```python
from build123d import *

# Parameters (mm, degrees)
F1_DEPTH = 1.905
F3_DEPTH = 1.905
F4_R     = 1.8415
F5_R     = 2.413
F6_DEPTH = 1.8415
F7_R     = 1.778
F8_W     = 81.534
F8_H     = 1.905
F9_DEPTH = 25.4
F10_R    = 5.08


with BuildPart() as f1:
    # F0 (on Top) → F1 (new body)
    with BuildSketch(Plane.XY):
        with BuildLine():
            Line((44.45, -15.875), (44.45, 15.875))
            Line((44.45, 15.875), (-44.45, 15.875))
            Line((-44.45, 15.875), (-44.45, -15.875))
            Line((-44.45, -15.875), (-25.4, -15.875))
            ThreePointArc((-25.4, -15.875), (-16.4197438789, -19.5947438789), (-12.7, -28.575))
            Line((-12.7, -28.575), (-12.7, -47.625))
            ThreePointArc((-12.7, -47.625), (0, -60.325), (12.7, -47.625))
            Line((12.7, -47.625), (12.7, -28.575))
            ThreePointArc((12.7, -28.575), (16.4197438789, -19.5947438789), (25.4, -15.875))
            Line((25.4, -15.875), (44.45, -15.875))
        make_face()
        with BuildLine():
            Line((5.1562, -22.3163515329), (5.1562, -47.625))
            ThreePointArc((5.1562, -47.625), (0, -52.7812), (-5.1562, -47.625))
            Line((-5.1562, -47.625), (-5.1562, -22.3163515329))
            ThreePointArc((-5.1562, -22.3163515329), (0, -17.1601515329), (5.1562, -22.3163515329))
        make_face(mode=Mode.SUBTRACT)
    extrude(amount=F1_DEPTH)

    # F2 (on face) → F3 (join)
    with BuildSketch(Plane(origin=(-44.45, 0, 0), x_dir=(0, -1, 0), z_dir=(-1, 0, 0))):
        with BuildLine():
            Line((-15.875, 41.275), (-15.875, 1.905))
            Line((-15.875, 1.905), (15.875, 1.905))
            Line((15.875, 1.905), (15.875, 41.275))
            Line((15.875, 41.275), (12.573, 41.275))
            ThreePointArc((12.573, 41.275), (5.5897728619, 30.0129056853), (-7.6027366345, 31.2610734641))
            ThreePointArc((-7.6027366345, 31.2610734641), (-8.0654902519, 34.6420492241), (-4.6845144919, 35.1048028415))
            ThreePointArc((-4.6845144919, 35.1048028415), (3.4442034806, 34.3357297657), (7.747, 41.275))
            Line((7.747, 41.275), (2.413, 41.275))
            ThreePointArc((2.413, 41.275), (0, 38.862), (-2.413, 41.275))
            Line((-2.413, 41.275), (-7.9572815939, 41.275))
            ThreePointArc((-7.9572815939, 41.275), (-10.0990117962, 39.9735577991), (-12.2407419985, 41.275))
            Line((-12.2407419985, 41.275), (-15.875, 41.275))
        make_face()
        with BuildLine():
            ThreePointArc((15.875, 41.275), (0, 57.15), (-15.875, 41.275))
            Line((-15.875, 41.275), (-12.2407419985, 41.275))
            ThreePointArc((-12.2407419985, 41.275), (-12.4710349135, 41.9437538571), (-12.4975270978, 42.6505527763))
            ThreePointArc((-12.4975270978, 42.6505527763), (-5.5381580453, 52.56256548), (6.5600004581, 52.0009835442))
            ThreePointArc((6.5600004581, 52.0009835442), (7.3595325655, 48.6834714629), (4.0420204843, 47.8839393555))
            ThreePointArc((4.0420204843, 47.8839393555), (-3.4124004118, 48.2299645887), (-7.7004964946, 42.1225628218))
            ThreePointArc((-7.7004964946, 42.1225628218), (-7.7896724982, 41.6869000206), (-7.9572815939, 41.275))
            Line((-7.9572815939, 41.275), (-2.413, 41.275))
            ThreePointArc((-2.413, 41.275), (0, 43.688), (2.413, 41.275))
            Line((2.413, 41.275), (7.747, 41.275))
            ThreePointArc((7.747, 41.275), (7.7353653871, 41.6994188123), (7.7004964946, 42.1225628218))
            ThreePointArc((7.7004964946, 42.1225628218), (9.8350168189, 44.7850731007), (12.4975270978, 42.6505527763))
            ThreePointArc((12.4975270978, 42.6505527763), (12.5541175954, 41.9638108593), (12.573, 41.275))
            Line((12.573, 41.275), (15.875, 41.275))
        make_face()
    extrude(amount=-F3_DEPTH)

    # F4
    f4_edges = [f1.edges().sort_by_distance(p)[0] for p in [
        (-44.45, 0, 0),
        (-42.545, 0, 1.905),
    ]]
    fillet(f4_edges, radius=F4_R)

    # F5 (on face) → F6 (join)
    with BuildSketch(Plane.YZ.offset(44.45)):
        with BuildLine():
            Line((-15.875, 41.3385), (-15.875, 1.905))
            Line((-15.875, 1.905), (-15.875, 0))
            Line((-15.875, 0), (15.875, 0))
            Line((15.875, 0), (15.875, 1.905))
            Line((15.875, 1.905), (15.875, 41.3385))
            ThreePointArc((15.875, 41.3385), (0, 57.2135), (-15.875, 41.3385))
        make_face()
        with BuildLine():
            ThreePointArc((-7.7672171262, 42.0276193774), (-3.8210671013, 34.5402395867), (4.6265424964, 35.0606704009))
            ThreePointArc((4.6265424964, 35.0606704009), (8.0006043661, 34.5499410208), (7.4898749861, 31.1758791512))
            ThreePointArc((7.4898749861, 31.1758791512), (-6.1858969034, 30.3333576051), (-12.5742896147, 42.4546206538))
            ThreePointArc((-12.5742896147, 42.4546206538), (-9.9572527322, 44.6446562598), (-7.7672171262, 42.0276193774))
        make_face(mode=Mode.SUBTRACT)
        with Locations((0, 41.3376752096)):
            Circle(F5_R, mode=Mode.SUBTRACT)
        with BuildLine():
            ThreePointArc((-6.3605039749, 52.2420007561), (5.8932381714, 52.5014590796), (12.591700736, 42.2373412666))
            ThreePointArc((12.591700736, 42.2373412666), (10.3568047712, 39.6585085798), (7.7779720844, 41.8934045446))
            ThreePointArc((7.7779720844, 41.8934045446), (3.6402899771, 48.2336141393), (-3.9289229785, 48.0733451146))
            ThreePointArc((-3.9289229785, 48.0733451146), (-7.2290412974, 48.9418824372), (-6.3605039749, 52.2420007561))
        make_face(mode=Mode.SUBTRACT)
    extrude(amount=-F6_DEPTH)

    # F7
    f7_edges = [f1.edges().sort_by_distance(p)[0] for p in [
        (44.45, 0, 0),
        (42.6085, 0, 1.905),
    ]]
    fillet(f7_edges, radius=F7_R)

    # F8 (on face) → F9 (join)
    with BuildSketch(Plane(origin=(0, 15.875, 0), x_dir=(-1, 0, 0), z_dir=(0, 1, 0))):
        with Locations((-0.0635, 0.9525)):
            Rectangle(F8_W, F8_H)
    extrude(amount=F9_DEPTH)

    # F10
    f10_edges = [f1.edges().sort_by_distance(p)[0] for p in [
        (40.8305, 41.275, 0.9525),
        (-40.7035, 41.275, 0.9525),
    ]]
    fillet(f10_edges, radius=F10_R)


solid = f1.part
```
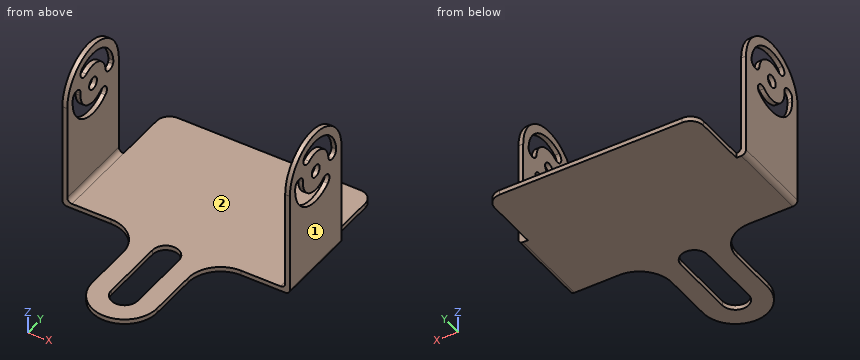
Check sheet for the modelled part. Datum: model origin and axes. Units: mm. Face numbers are marked on the shaded views. A direction names the side the tool comes from. Give positions to 0.01 mm unless a question says otherwise; leave off trailing zeros. Order: outer loops, then holes, each group sorted by start corner. A loop starts at its lowest first (then second) coordinate and runs counter-clockwise, first axis right, second up. Notation, with made-up numbers: M 11.25,4.25 L 39.25,4.25 A8 cw 39.25,12.25 Z; hole C 65.5,85.25 d2. An arc over 180 degrees is marked long. Answer in a Markdown table with one row per item. Add a question column.
Q1. Thickness scan on L1, parallel to Z at x = -43.95, y = 0; L2, parallel to Z at x = 43.55, y = 0; L3, parallel to Z at x = 11, y = 19 (3 decimals). Record the ranges inside material, lowest first.
Q2. Access from +Z, -Z, +X, -X, +Y, -Y to the whole of each face (thin tool, end or side, straight path). Record for the marked faces 1 and 2.
Q3. Gauge pin test, flat ends, axial feed: pin 1 Ø5.5 at (x, z) = (-37.5, 24) entering from -Y; pin 2 Ø1.5 at (y, z) = (22, 1) entering from +X; pin 3 Ø24.5 at (x, y) = (6.5, 4.5) entering from +Z (3 decimals); pin 4 Ø0.6 at (y, z) = (22.5, 0.5) entering from -X. Record the tip position at first contact, or that the pin passes through.
Q4. Sectioned sample at C-C, the plane y = -11. Count the separate pieces of the cut face and the enclosed holes in it, and give its area (3 significant figures).
Q5. Sectioned sample at B-B, the plane x = 0. Record the boundary of the cut face in (y, z) (3 decimals).
Verdict:
| question | item | result |
|---|---|---|
| 1 | L1 | 0.58 to 28.7, 33.53 to 38.86, 43.69 to 49.02, 53.85 to 57.15 |
| 1 | L2 | 0.23 to 28.71, 33.54 to 38.92, 43.75 to 49.14, 53.96 to 57.21 |
| 1 | L3 | 0 to 1.905 |
| 2 | face 1 | +Z, -Z, +X, +Y, -Y |
| 2 | face 2 | +Z, +Y, -Y |
| 3 | pin 1 | through |
| 3 | pin 2 | x = 40.83 |
| 3 | pin 3 | z = 1.905 |
| 3 | pin 4 | x = -40.7 |
| 4 | separate pieces | 3 |
| 4 | enclosed holes | 0 |
| 4 | area | 325 mm² |
| 5 | outline | M -60.325,0 L -52.781,0 L -52.781,1.905 L -60.325,1.905 Z; M -17.16,0 L 41.275,0 L 41.275,1.905 L -17.16,1.905 Z |
